```python
from build123d import *

# Parameters (mm, degrees)
F1_DEPTH = 7


with BuildPart() as f1:
    # F0 (on Top) → F1 (new body)
    with BuildSketch(Plane.XY):
        with BuildLine():
            ThreePointArc((7.5680259261, 8.0172070312), (10.1239347794, 4.3653830969), (11.025, 0))
            ThreePointArc((11.025, 0), (10.1239347794, -4.3653830969), (7.5680259261, -8.0172070312))
            ThreePointArc((7.5680259261, -8.0172070313), (8.8929301367, -9.5257592273), (9.9215674165, -11.25))
            ThreePointArc((9.9215674165, -11.25), (13.6715674165, -6.1715674165), (15, 0))
            ThreePointArc((15, 0), (13.6715674165, 6.1715674165), (9.9215674165, 11.25))
            ThreePointArc((9.9215674165, 11.25), (8.8929301367, 9.5257592273), (7.5680259261, 8.0172070312))
        make_face()
        with BuildLine():
            ThreePointArc((5.5250997211, 9.5406445313), (6.5907283556, 8.8381516587), (7.5680259261, 8.0172070312))
            ThreePointArc((7.5680259261, 8.0172070312), (8.8929301367, 9.5257592273), (9.9215674165, 11.25))
            ThreePointArc((9.9215674165, 11.25), (8.9252455049, 12.0557037405), (7.863796439, 12.7734375))
            ThreePointArc((7.863796439, 12.7734375), (6.8868260245, 11.0178691999), (5.5250997211, 9.5406445312))
        make_face()
        with BuildLine():
            ThreePointArc((9.9215674165, -11.25), (8.8929301367, -9.5257592273), (7.5680259261, -8.0172070313))
            ThreePointArc((7.5680259261, -8.0172070312), (6.5907283556, -8.8381516587), (5.5250997211, -9.5406445313))
            ThreePointArc((5.5250997211, -9.5406445312), (6.8868260245, -11.0178691999), (7.863796439, -12.7734375))
            ThreePointArc((7.863796439, -12.7734375), (8.9252455049, -12.0557037405), (9.9215674165, -11.25))
        make_face()
        with BuildLine():
            ThreePointArc((7.863796439, 12.7734375), (8.9252455049, 12.0557037405), (9.9215674165, 11.25))
            ThreePointArc((9.9215674165, 11.25), (10.7270042785, 13.5645576974), (11, 16))
            ThreePointArc((11, 16), (7.7781745931, 23.7781745931), (0, 27))
            Line((0, 27), (0, 24.5))
            ThreePointArc((0, 24.5), (6.0104076401, 22.0104076401), (8.5, 16))
            ThreePointArc((8.5, 16), (8.3394325266, 14.3556566252), (7.863796439, 12.7734375))
        make_face()
        with BuildLine():
            ThreePointArc((11, -16), (10.7270042785, -13.5645576974), (9.9215674165, -11.25))
            ThreePointArc((9.9215674165, -11.25), (8.9252455049, -12.0557037405), (7.863796439, -12.7734375))
            ThreePointArc((7.863796439, -12.7734375), (8.3394325266, -14.3556566252), (8.5, -16))
            ThreePointArc((8.5, -16), (6.0104076401, -22.0104076401), (0, -24.5))
            Line((0, -24.5), (0, -27))
            ThreePointArc((0, -27), (7.7781745931, -23.7781745931), (11, -16))
        make_face()
        with BuildLine():
            ThreePointArc((-9.9215674165, 11.25), (-8.8929301367, 9.5257592273), (-7.5680259261, 8.0172070313))
            ThreePointArc((-7.5680259261, 8.0172070312), (-6.5907283556, 8.8381516587), (-5.5250997211, 9.5406445313))
            ThreePointArc((-5.5250997211, 9.5406445312), (-6.8868260245, 11.0178691999), (-7.863796439, 12.7734375))
            ThreePointArc((-7.863796439, 12.7734375), (-8.9252455049, 12.0557037405), (-9.9215674165, 11.25))
        make_face()
        with BuildLine():
            ThreePointArc((-7.5680259261, -8.0172070312), (-11.025, 0), (-7.5680259261, 8.0172070312))
            ThreePointArc((-7.5680259261, 8.0172070313), (-8.8929301367, 9.5257592273), (-9.9215674165, 11.25))
            ThreePointArc((-9.9215674165, 11.25), (-15, 0), (-9.9215674165, -11.25))
            ThreePointArc((-9.9215674165, -11.25), (-8.8929301367, -9.5257592273), (-7.5680259261, -8.0172070313))
        make_face()
        with BuildLine():
            ThreePointArc((-5.5250997211, -9.5406445313), (-6.5907283556, -8.8381516587), (-7.5680259261, -8.0172070312))
            ThreePointArc((-7.5680259261, -8.0172070313), (-8.8929301367, -9.5257592273), (-9.9215674165, -11.25))
            ThreePointArc((-9.9215674165, -11.25), (-8.9252455049, -12.0557037405), (-7.863796439, -12.7734375))
            ThreePointArc((-7.863796439, -12.7734375), (-6.8868260245, -11.0178691999), (-5.5250997211, -9.5406445312))
        make_face()
        with BuildLine():
            ThreePointArc((0, 27), (-9.3072552345, 21.8630196998), (-9.9215674165, 11.25))
            ThreePointArc((-9.9215674165, 11.25), (-8.9252455049, 12.0557037405), (-7.863796439, 12.7734375))
            ThreePointArc((-7.863796439, 12.7734375), (-7.0595956417, 20.7341429399), (0, 24.5))
            Line((0, 24.5), (0, 27))
        make_face()
        with BuildLine():
            ThreePointArc((-9.9215674165, -11.25), (-9.3072552345, -21.8630196998), (0, -27))
            Line((0, -27), (0, -24.5))
            ThreePointArc((0, -24.5), (-7.0595956417, -20.7341429399), (-7.863796439, -12.7734375))
            ThreePointArc((-7.863796439, -12.7734375), (-8.9252455049, -12.0557037405), (-9.9215674165, -11.25))
        make_face()
    extrude(amount=F1_DEPTH)


solid = f1.part
```
The listing builds one solid part. Answer for the finished solid, in the listing's coordinates (mm). Give positions to 0.01 mm unless a question says otherwise; leave off trailing zeros. Order: outer loops, then holes, each group sorted by start corner. A loop starts at its lowest first (then second) coordinate and runs counter-clockwise, first axis right, second up. Notation, with made-up numbers: (46.25, 62.25) - (68.25, 62.25) arc R18 cw to (68.25, 97.25) - close; hole circle Ø9 at (17, 48.5). An arc over 180 degrees is marked (long way). Use one line per item in the form item = value. Start each with the question number.
(1) Flat-ended cylindrical pins translate along their axes: pin 1 Ø13.5 at (x, y) = (0, -16) entering from +Z; pin 2 Ø3 at (x, z) = (-5.5, 5) entering from -Y; pin 3 Ø1.5 at (x, z) = (-9.5, 6) entering from +Y. Find the tip coordinate at first contact, or state that the pin passes through.
(2) A cutting plane is placed at A-A, the plane y = -14. Write down the section's boundary in (x, z).
(3) A cutting plane is placed at C-C, the plane x = 5. Write down the section's boundary in (y, z), then the cut area to 3 significant figures.
(4) A cutting plane is placed at B-B, the plane z = 3.75. Write down the section's boundary in (x, y) (3 decimals).
(5) Consider line 1 (X direction, y = 0.5, z = 0.75); line 2 (Y direction, x = 10, z = 1.5); line 3 (X direction, y = -16, z = 4.75). Determine where each line is inside the solid, lowest interval first. Write a range as from..to.
Ans:
q1.pin_1 = through
q1.pin_2 = -26.25
q1.pin_3 = 22.67
q2.outline = (-10.82, 0) - (-8.26, 0) - (-8.26, 7) - (-10.82, 7) - close; (8.26, 0) - (10.82, 0) - (10.82, 7) - (8.26, 7) - close
q3.outline = (-25.8, 0) - (-22.87, 0) - (-22.87, 7) - (-25.8, 7) - close; (22.87, 0) - (25.8, 0) - (25.8, 7) - (22.87, 7) - close
q3.area = 40.9 mm^2
q4.outline = (-9.922, -11.25) arc R11 ccw (long way) to (9.922, -11.25) arc R15 ccw to (9.922, 11.25) arc R11 ccw (long way) to (-9.922, 11.25) arc R15 ccw to start; hole (-5.525, -9.541) arc R8.5 ccw (long way) to (5.525, -9.541) arc R11.025 ccw to (5.525, 9.541) arc R8.5 ccw (long way) to (-5.525, 9.541) arc R11.025 ccw to start
q5.line_1 = -14.99..-11.01, 11.01..14.99
q5.line_2 = -20.58..-11.42, -11.18..-4.64, 4.64..11.18, 11.42..20.58
q5.line_3 = -11..-8.5, 8.5..11
